Build history of the part. All positions in model axes, mm. A direction names the side the tool comes from. Coordinates: 2 decimals unless noted, no trailing zeros. Order: outer loops, then holes, each group sorted by start corner. A loop starts at its lowest first (then second) coordinate and runs counter-clockwise, first axis right, second up. Notation, with made-up numbers: (-15, 47) - (41, 47) arc R18 cw to (41, 73) - close; hole circle Ø5 at (67.5, 29.5). An arc over 180 degrees is marked (long way). Write each question's results on one line, items separated by ' | '.
Autodesk Inventor part; units mm, degrees
ref_plane "YZ Plane" through (0, 0, 0) normal (1, 0, 0) x (0, 1, 0)
ref_plane "XZ Plane" through (0, 0, 0) normal (0, 1, 0) x (-1, 0, 0)
ref_plane "XY Plane" through (0, 0, 0) normal (0, 0, 1) x (1, 0, 0)
sketch "Skizze1" plane through (0, 0, 0) normal (1, 0, 0) x (0, 1, 0)
  circle A0 centre (7.8808, 0) radius 5
  circle A1 centre (-9.6192, 0) radius 8.5
  arc A2 (-6.8769, 8.0455) -> (8.2347, 4.9875) centre (12.4808, 64.837) ccw
  arc A3 (8.2347, -4.9875) -> (-6.8769, -8.0455) centre (12.4808, -64.837) ccw
  point P0 (0, 0)
  dimension "d0" = 10
  dimension "d1" = 17
  dimension "d2" = 17.5
  dimension "d3" = 60
  dimension "d4" = 0
  dimension "d5" = 0
  dimension "d6" = 60
extrude "Extrusion1" add sketch "Skizze1" along normal blind 8
sketch "Skizze2" plane through (8, 0, 0) normal (1, 0, 0) x (0, 0, -1)
  arc A0 (4.9875, 8.2347) -> (-4.9875, 8.2347) centre (0, 7.8808) ccw
  circle A1 centre (0, 7.8808) radius 4.1
  point P0 (0, 0)
  dimension "d9" = 8.2
extrude "Extrusion2" add sketch "Skizze2" along normal blind 10
sketch "Skizze4" plane through (0, 0, 0) normal (-1, 0, 0) x (0, 0, 1)
  arc A0 (-8.0455, -6.8769) -> (8.0455, -6.8769) centre (0, -9.6192) ccw
  line L0 (-6.9859, -9.6192) -> (-3.493, -3.5692)
  line L1 (-3.493, -3.5692) -> (3.493, -3.5692)
  line L2 (3.493, -3.5692) -> (6.9859, -9.6192)
  line L3 (6.9859, -9.6192) -> (3.493, -15.6692)
  line L4 (3.493, -15.6692) -> (-3.493, -15.6692)
  line L5 (-3.493, -15.6692) -> (-6.9859, -9.6192)
  point P0 (0, 0)
  dimension "d15" = 12.1
extrude "Extrusion4" cut sketch "Skizze4" against normal blind 6
properties part number "MotorAnkerNeu"
1. Drop flat-ended pins along their axis: pin 1 Ø3 at (x, z) = (3.5, -0.5) entering from -Y; pin 2 Ø2 at (x, z) = (2.5, -2.5) entering from -Y; pin 3 Ø6 at (y, z) = (-11.5, 0.5) entering from -X; pin 4 Ø4 at (y, z) = (-6.5, 2.5) entering from +X. Give the stop position or say it passes through.
Solved:
pin 1: stops at y = -18.12 | pin 2: stops at y = -17.99 | pin 3: stops at x = 6 | pin 4: stops at x = 8
2. Band-saw the part on B-B on x = 4.75. Give the cut face in (y, z).
Solved:
outline: (-6.88, -8.05) arc R60 cw to (8.23, -4.99) arc R5 ccw to (8.23, 4.99) arc R60 cw to (-6.88, 8.05) arc R8.5 ccw (long way) to start; hole (-15.67, -3.49) - (-9.62, -6.99) - (-3.57, -3.49) - (-3.57, 3.49) - (-9.62, 6.99) - (-15.67, 3.49) - close
3. Band-saw the part on D-D on y = -4. Give the cut face in (x, z), then the cut area to 3 significant figures.
Solved:
outline: (0, -7.14) - (8, -7.14) - (8, 7.14) - (0, 7.14) - (0, 3.74) - (6, 3.74) - (6, -3.74) - (0, -3.74) - close | area: 69.4 mm2
4. Probe line 1 (X direction, y = -9.5, z = 4); line 2 (X direction, y = 7, z = -4.5); line 3 (Y direction, x = 5.25, z = 2.5). List the from-to ranges inside material, lowest first.
Solved:
line 1: x = 6 to 8 | line 2: x = 0 to 8 | line 3: y = -17.74 to -15.67, -3.57 to 12.21
5. Band-saw the part on C-C on y = 6. Give the cut face in (x, z).
Solved:
outline: (0, -5.19) - (8, -5.19) - (8, -3.64) - (18, -3.64) - (18, 3.64) - (8, 3.64) - (8, 5.19) - (0, 5.19) - close
6. Two-plate mould, pull along Y, no slides. Class faces 1 (the face through (2.958, -6.637, -5.264)), 2 (the face through (8, -6, 0)), 3 (the face through (12.93, 3.816, 0.534)): +Y half, -Y half, draft (parallel to the pull), parting line (faces both ways), or undercut.
Solved:
face 1: undercut | face 2: draft | face 3: parting line
7. Tool access for faces 4 (the face through (2.958, -12.602, 5.264)), 5 (the face through (0, -3, 0)): list every direction of +Z, -Z, +X, -X, +Y, -Y with a clear straight run to the whole face (end or side of a thin tool).
Solved:
face 4: -X | face 5: +Z, -Z, -X, +Y, -Y
8. Band-saw the part on A-A on z = 0. Give the cut face in (x, y).
Solved:
outline: (0, -18.12) - (8, -18.12) - (8, 3.78) - (18, 3.78) - (18, 11.98) - (8, 11.98) - (8, 12.88) - (0, 12.88) - (0, -3.57) - (6, -3.57) - (6, -15.67) - (0, -15.67) - close
